Build history of the part. All positions in model axes, mm. Face numbers are marked on the shaded views. A direction names the side the tool comes from. Round coordinates to 2 decimals unless told otherwise and drop trailing zeros. Write each loop counter-clockwise with the first axis right and the second up, starting at its lowest first coordinate (ties: lowest second). Pieces come first, ordered by that corner, then holes.
Item 1: Drop flat-ended pins along their axis: pin 1 Ø1.5 at (x, y) = (20, 30) entering from +Z; pin 2 Ø3 at (y, z) = (47, 39) entering from +X; pin 3 Ø1 at (x, y) = (27, 68) entering from -Z. Give the stop position or say it passes through.
Item 2: 3-axis set-ups, long thin cutter, end or side, ignore diameter. For the marked faces 1, 2 and 3: which of +Z, -Z, +X, -X, +Y, -Y reach the whole face in a straight line?
Item 3: Mould opens along Z. For the marked faces 4, 5 and 6 say: +Z half, -Z half, draft (parallel to the pull), parting line (faces both ways), or undercut.
Item 4: Band-saw the part on A-A, the plane y = 78. Write the cut outline in (x, z).
Item 5: Wall check: probe 1 along Z at (x, y) = (2.5, 11); probe 2 along Z at (x, y) = (19.78, 15); probe 3 along Z at (x, y) = (0, 22.5). Give the ranges that are in metal, low to high.
Item 6: Band-saw the part on D-D, the plane z = -48.5. Write the cut outline in (x, y), then the cut area to 3 significant figures.
Item 7: Band-saw the part on B-B, the plane z = 0. Write the cut outline in (x, y), then the cut area to 3 significant figures.
Item 8: Band-saw the part on C-C, the plane y = 23.5. Write the cut outline in (x, z).
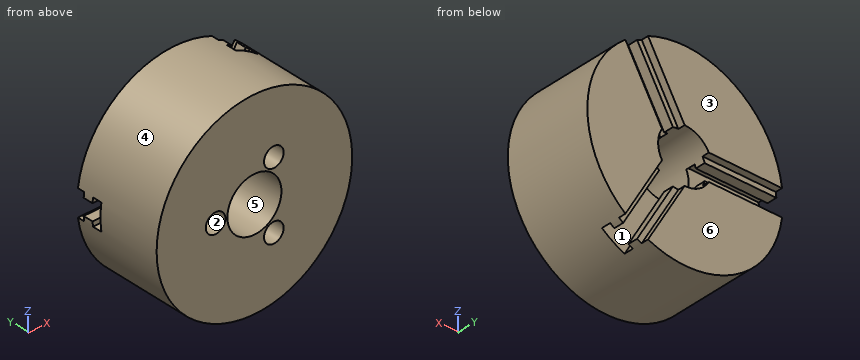
Autodesk Inventor part; units mm, degrees
ref_plane "XZ Plane" through (0, 0, 0) normal (0, 1, 0) x (-1, 0, 0)
ref_plane "XY Plane" through (0, 0, 0) normal (0, 0, 1) x (1, 0, 0)
sketch "Sketch1" plane through (0, 0, 0) normal (0, 1, 0) x (-1, 0, 0)
  circle A0 centre (0, 0) radius 99.7
extrude "Extrusion1" add sketch "Sketch1" along normal blind 90.9
sketch "Sketch2" plane through (0, 90.9, 0) normal (0, 1, 0) x (1, 0, 0)
  circle A0 centre (0, 0) radius 27.56
  dimension "d3" = 55.12
extrude "Extrusion2" cut sketch "Sketch2" against normal blind 90.9
sketch "Sketch3" plane through (0, 90.9, 0) normal (0, 1, 0) x (1, 0, 0)
  circle A0 centre (0, 0) radius 99.7
  line L0 (-99.7, 0) -> (-98.8062, 13.32)
  line L1 (-98.8062, 13.32) -> (-24.1274, 13.32)
  circle A1 centre (0, 0) radius 27.56
  line L2 (-99.7, 0) -> (-98.8062, -13.32)
  line L3 (-98.8062, -13.32) -> (-24.1274, -13.32)
  line L4 (37.8676, -92.2287) -> (0.5282, -27.5549)
  line L5 (49.85, -86.3427) -> (37.8676, -92.2287)
  line L6 (49.85, -86.3427) -> (60.9386, -78.9087)
  line L7 (60.9386, -78.9087) -> (23.5992, -14.2349)
  line L8 (60.9386, 78.9087) -> (23.5992, 14.2349)
  line L9 (49.85, 86.3427) -> (60.9386, 78.9087)
  line L10 (49.85, 86.3427) -> (37.8676, 92.2287)
  line L11 (37.8676, 92.2287) -> (0.5282, 27.5549)
  line L12 (-24.1274, 13.32) -> (-24.1274, -13.32)
  line L13 (0.5282, 27.5549) -> (23.5992, 14.2349)
  line L14 (23.5992, -14.2349) -> (0.5282, -27.5549)
  dimension "d6" = 13.35
  dimension "d15" = 360
extrude "Extrusion6" cut sketch "Sketch3" against normal blind 7.18 contours L8 A1 L11 L10 L9 | L6 L5 L4 A1 L7 | L13 A1 | A1 L14 | L1 A1 L3 L2 L0
sketch "Sketch7" plane through (49.85, 83.72, -86.3427) normal (-0.5569, 0, 0.8306) x (0.8306, 0, 0.5569)
  line L0 (13.35, 7.18) -> (0, 7.18)
  line L1 (13.35, 0) -> (13.35, 7.18)
  line L2 (0, 7.18) -> (13.35, 7.18)
  line L3 (13.35, 0) -> (18.3498, 0)
  line L4 (13.35, 7.18) -> (13.35, 0)
  line L5 (0, 7.18) -> (0, 0)
  line L6 (13.35, 0) -> (0, 0)
  line L7 (0, 0) -> (0, 6.2119)
  line L8 (0, 7.18) -> (-13.2303, 7.18)
  line L9 (-13.2303, 4.6736) -> (0, 7.18)
  line L10 (0, 7.18) -> (0, 0)
  line L11 (-13.2303, -2.9965) -> (-13.2303, 4.6736)
  line L12 (-13.2303, 0) -> (-13.2303, 7.18)
  point P0 (6.675, -83.72)
extrude "Extrusion7" cut sketch "Sketch7" against normal blind 10 contours L1 L6 L5 L0
sketch "Sketch8" plane through (37.8676, 83.72, -92.2287) normal (-0.4409, 0, 0.8976) x (0.8976, 0, 0.4409)
  line L0 (0, 0) -> (0, 7.18)
  line L1 (-4.9998, 0) -> (0, 0)
  line L2 (0, 7.18) -> (0, 0)
  line L3 (0, 0) -> (13.35, 0)
  line L4 (0, 0) -> (13.35, 0)
  line L5 (13.35, 7.18) -> (13.35, 0)
  line L6 (13.35, 0) -> (13.35, 7.18)
  line L7 (0, 7.18) -> (13.35, 7.18)
  line L8 (13.35, 7.18) -> (0, 7.18)
  line L9 (0, 7.18) -> (0, 4.7035)
  point P0 (6.675, -83.72)
extrude "Extrusion8" cut sketch "Sketch8" against normal blind 10
sketch "Sketch10" plane through (49.85, 83.72, 86.3427) normal (-0.4409, 0, -0.8976) x (-0.8976, 0, 0.4409)
  line L0 (0, 7.18) -> (13.35, 7.18)
  line L1 (13.35, 7.18) -> (18.3498, 7.18)
  line L2 (0, 7.18) -> (13.35, 7.18)
  line L3 (13.35, 0) -> (18.3498, 0)
  line L4 (13.35, 7.18) -> (13.35, 0)
  line L5 (0, 0) -> (13.35, 0)
  line L6 (13.35, 0) -> (0, 0)
  line L7 (0, 0) -> (0, 7.18)
  line L8 (0, 7.18) -> (0, 0)
  point P0 (6.675, -83.72)
extrude "Extrusion9" cut sketch "Sketch10" against normal blind 10
sketch "Sketch11" plane through (60.9386, 83.72, 78.9087) normal (-0.5569, 0, -0.8306) x (-0.8306, 0, 0.5569)
  line L0 (-4.9998, 7.18) -> (0, 7.18)
  line L1 (96.1615, 7.18) -> (0, 7.18)
  line L2 (0, 7.18) -> (13.35, 7.18)
  line L3 (0, 0) -> (13.35, 0)
  line L4 (13.35, 7.18) -> (13.35, 0)
  line L5 (13.35, 0) -> (0, 0)
  line L6 (0, 0) -> (0, 7.18)
  line L7 (0, 0) -> (0, 7.18)
  point P0 (6.675, -83.72)
extrude "Extrusion10" cut sketch "Sketch11" against normal blind 10
sketch "Sketch12" plane through (0, 90.9, 0) normal (0, 1, 0) x (1, 0, 0)
  arc A0 (37.8676, -92.2287) -> (60.9386, -78.9087) centre (0, 0) ccw
  arc A1 (-99.7, 0) -> (-98.8062, -13.32) centre (0, 0) ccw
  arc A2 (60.9386, 78.9087) -> (37.8676, 92.2287) centre (0, 0) ccw
  circle A3 centre (0, 0) radius 99.7
  arc A4 (-98.8062, -13.32) -> (37.8676, -92.2287) centre (0, 0) ccw
  arc A5 (-98.8062, 13.32) -> (-99.7, 0) centre (0, 0) ccw
  arc A6 (37.8676, 92.2287) -> (-98.8062, 13.32) centre (0, 0) ccw
  arc A7 (60.9386, -78.9087) -> (60.9386, 78.9087) centre (0, 0) ccw
  point P0 (-99.7, 0)
sketch "Sketch13" plane through (0, 83.72, 0) normal (0, 1, 0) x (1, 0, 0)
  arc A0 (60.9386, 78.9087) -> (37.8676, 92.2287) centre (0, 0) ccw
ref_plane "Work Plane10" through (-99.7, 0, 0) normal (1, 0, 0) x (0, 1, 0)
sketch "Sketch16" plane through (-99.7, 0, 0) normal (1, 0, 0) x (0, 1, 0)
  line L0 (83.72, 0) -> (83.72, -13.32)
  line L1 (83.72, -8.22) -> (73.62, -8.22)
  line L2 (83.72, 13.32) -> (83.72, 0)
  line L3 (83.72, 8.22) -> (73.62, 8.22)
  line L4 (73.62, -8.22) -> (73.62, -13.32)
  line L5 (73.62, -13.32) -> (64.1, -13.32)
  line L6 (64.1, -13.32) -> (64.1, 13.32)
  line L7 (64.1, 13.32) -> (73.62, 13.32)
  line L8 (73.62, 13.32) -> (73.62, 8.22)
  line L9 (83.72, -8.22) -> (83.72, 8.22)
  point P0 (0, 0)
  dimension "d36" = 9.52
extrude "Extrusion11" cut sketch "Sketch16" along normal blind 74.5875
sketch "Sketch18" plane through (-98.8062, 83.72, -13.32) normal (0.9978, 0, 0.067) x (0.067, 0, -0.9978)
  line L0 (0, 0) -> (0, 7.18)
  line L1 (0, 7.18) -> (0, 0)
  arc A0 (0, 0) -> (-2.79, 0) centre (-1.395, 0) ccw
  line L2 (-13.35, 0) -> (-21.5289, 0)
  line L3 (-2.79, 0) -> (-13.35, 0)
  arc A1 (-13.35, 2.7204) -> (-13.35, 0) centre (-13.35, 1.3602) ccw
  line L4 (-13.35, 2.7204) -> (-13.35, 7.18)
  line L5 (-19.298, 7.18) -> (9.1079, 7.18)
  point P0 (-6.675, -83.72)
extrude "Extrusion12" cut sketch "Sketch18" along normal blind 74.5875
sketch "Sketch20" plane through (-99.7, 0, 0) normal (1, 0, 0) x (0, 1, 0)
  line L0 (90.9, 0) -> (90.9, -13.32)
  line L1 (83.72, -13.32) -> (90.9, -13.32)
  line L2 (90.9, -13.32) -> (83.72, -13.32)
  line L3 (83.72, 8.22) -> (83.72, 13.32)
  line L4 (83.72, -13.32) -> (83.72, 13.32)
  line L5 (83.72, 13.32) -> (90.9, 13.32)
  line L6 (90.9, 13.32) -> (90.9, -13.32)
  point P0 (0, 0)
extrude "Extrusion13" cut sketch "Sketch20" along normal blind 10
pattern_circular "Circular Pattern1" count 3 over 360 about axis through (0, 90.9, 0) along (0, -1, 0) of "Extrusion11"
sketch "Sketch21" plane through (0, 0, 0) normal (0, -1, 0) x (1, 0, 0)
  arc A0 (-98.8062, -13.32) -> (37.8676, -92.2287) centre (0, 0) ccw
  circle A1 centre (-39.56, 0) radius 10
  circle A2 centre (19.78, -34.26) radius 10
  circle A3 centre (19.78, 34.26) radius 10
  point P0 (-25.1125, 13.32)
  dimension "d50" = 360
extrude "Extrusion14" cut sketch "Sketch21" against normal blind 50
properties part number "3 jaww" material "Steel"
Results:
1. pin 1: stops at z = 97.82
1. pin 2: stops at x = 92.38
1. pin 3: stops at z = -96.11
2. face 1: none
2. face 2: -Y
2. face 3: +Z, -Z, +X, -X, +Y
3. face 4: parting line
3. face 5: undercut
3. face 6: draft
4. outline: (-99.36, -8.22) arc R99.7 ccw to (42.56, -90.16) - (6.03, -26.89) arc R27.56 cw to (-26.31, -8.22) - close; (-99.36, 8.22) - (-26.31, 8.22) arc R27.56 cw to (6.03, 26.89) - (42.56, 90.16) arc R99.7 ccw to start; (20.27, -18.67) - (56.8, -81.94) arc R99.7 ccw to (56.8, 81.94) - (20.27, 18.67) arc R27.56 cw to start
5. probe 1: z = -99.67 to -27.45, 27.45 to 99.67
5. probe 2: z = -97.72 to -44.26, -24.26 to -19.19, 19.19 to 24.26, 44.26 to 97.72
5. probe 3: z = -99.7 to -27.56, 27.56 to 99.7
6. outline: (-87.11, 0) - (87.11, 0) - (87.11, 90.9) - (43.38, 90.9) - (43.38, 83.72) - (37.49, 83.72) - (37.49, 73.62) - (43.38, 73.62) - (43.38, 64.1) - (12.62, 64.1) - (12.62, 73.62) - (18.51, 73.62) - (18.51, 83.72) - (12.62, 83.72) - (12.62, 90.9) - (-87.11, 90.9) - close
6. area: 15,100 mm2
7. outline: (-99.7, 0) - (-49.56, 0) - (-49.56, 50) - (-29.56, 50) - (-29.56, 0) - (-27.56, 0) - (-27.56, 64.1) - (-99.7, 64.1) - close; (27.56, 0) - (99.7, 0) - (99.7, 90.9) - (27.56, 90.9) - close
7. area: 10,200 mm2
8. outline: circle Ø199.4 at (0, 0); hole circle Ø20 at (-39.56, 0); hole circle Ø55.12 at (0, 0); hole circle Ø20 at (19.78, -34.26); hole circle Ø20 at (19.78, 34.26)
